Geometry check sheet. Reference: the model listing, model coordinates, mm. A direction names the side the tool comes from. Round coordinates to 2 decimals unless told otherwise and drop trailing zeros. Loops run counter-clockwise (first coordinate to the right, second up) from the corner with the lowest first, then second, coordinate; pieces in that order, holes last. Notation, with made-up numbers: (45.5, 29) - (101.5, 29) arc R21 cw to (101.5, 68) - close; hole circle Ø4 at (-11.5, 64). An arc over 180 degrees is marked (long way). Write item = value, one per line.
```python
from build123d import *

# Parameters (mm, degrees)
SKETCH1_W                = 98
SKETCH1_H                = 90
BOSS_EXTRUDE1_DEPTH      = 15
CUT_EXTRUDE1_DEPTH       = 15
CUT_EXTRUDE2_DEPTH       = 15
CUT_EXTRUDE5_DEPTH       = 100
CUT_EXTRUDE6_DEPTH       = 100
SKETCH9_R                = 9.5
CUT_EXTRUDE7_DEPTH       = 45
SKETCH10_R               = 9.5
CUT_EXTRUDE8_DEPTH       = 45
BOSS_EXTRUDE3_DEPTH      = 100
BOSS_EXTRUDE4_DEPTH      = 100
SKETCH14_W               = 54.537944566
SKETCH14_H               = 37.433727788
CUT_EXTRUDE9_DEPTH       = 100
SKETCH15_W               = 37.221464136
SKETCH15_H               = 31.979004399
CUT_EXTRUDE10_DEPTH      = 100
BOSS_EXTRUDE5_DEPTH      = 15
BOSS_EXTRUDE6_DEPTH      = 15
BOSS_EXTRUDE7_DEPTH      = 15
CUT_EXTRUDE11_DEPTH      = 100
SKETCH20_R               = 9.5
CUT_EXTRUDE12_DEPTH      = 45
SKETCH21_R               = 9.5
CUT_EXTRUDE13_DEPTH      = 100
SKETCH22_R               = 9.5
BOSS_EXTRUDE8_DEPTH      = 55
SKETCH23_R               = 9.5
CUT_EXTRUDE14_DEPTH      = 55
SKETCH24_R               = 9.5
CUT_EXTRUDE15_DEPTH      = 100
SKETCH25_R               = 9.5
BOSS_EXTRUDE10_DEPTH     = 100
SKETCH26_R               = 9.5
CUT_EXTRUDE16_DEPTH      = 100
SKETCH27_W               = 176.377882562
SKETCH27_H               = 122.842530298
SKETCH27_W_2             = 98
SKETCH27_H_2             = 90
CUT_EXTRUDE19_DEPTH      = 100
CUT_EXTRUDE19_DEPTH_BACK = 100
SKETCH28_W               = 109.510814303
SKETCH28_H               = 24.111992001
CUT_EXTRUDE20_DEPTH      = 100
SKETCH29_R               = 9.59940523
CUT_EXTRUDE21_DEPTH      = 100
SKETCH30_W               = 22
SKETCH30_H               = 32
CUT_EXTRUDE22_DEPTH      = 100
SKETCH31_W               = 16.2
SKETCH31_H               = 12
CUT_EXTRUDE23_DEPTH      = 100
CUT_EXTRUDE24_DEPTH      = 13
SKETCH33_W               = 50.373016546
SKETCH33_H               = 2
BOSS_EXTRUDE12_DEPTH     = 15
SKETCH34_W               = 20
SKETCH34_H               = 2
CUT_EXTRUDE25_DEPTH      = 5
CUT_EXTRUDE27_DEPTH      = 100
SKETCH37_W               = 14
SKETCH37_H               = 11
CUT_EXTRUDE28_DEPTH      = 13
CUT_EXTRUDE32_DEPTH      = 9.5


with BuildPart() as part:
    # Sketch1 → Boss-Extrude1 (new body)
    with BuildSketch(Plane(origin=(0, 0, 0), x_dir=(1, 0, 0), z_dir=(0, 1, 0))):
        with Locations((7.915679061, -25.165675541)):
            Rectangle(SKETCH1_W, SKETCH1_H)
    extrude(amount=BOSS_EXTRUDE1_DEPTH)

    # Sketch3 → Cut-Extrude1 (cut)
    with BuildSketch(Plane(origin=(0, 15, 0), x_dir=(1, 0, 0), z_dir=(0, 1, 0))):
        Polygon((-41.084320939, -35.165675541), (-6.084320939, -70.165675541), (-41.084320939, -70.165675541), align=None)
        Polygon((21.915679061, -70.165675541), (56.915679061, -35.165675541), (56.915679061, -70.165675541), align=None)
    extrude(amount=-CUT_EXTRUDE1_DEPTH, mode=Mode.SUBTRACT)

    # Sketch4 → Cut-Extrude2 (cut)
    with BuildSketch(Plane(origin=(0, 15, 0), x_dir=(1, 0, 0), z_dir=(0, 1, 0))):
        Polygon((-41.084320939, -35.165675541), (-32.241899351, -26.323253953), (-41.084320939, -17.480832365), align=None)
        Polygon((56.915679061, -17.480832365), (48.073257473, -26.323253953), (56.915679061, -35.165675541), align=None)
    extrude(amount=-CUT_EXTRUDE2_DEPTH, mode=Mode.SUBTRACT)

    # Sketch5 → Cut-Extrude5 (cut)
    with BuildSketch(Plane(origin=(-2.959322699, 0, -2.959322699), x_dir=(-0.707106781, 0, 0.707106781), z_dir=(-0.707106781, 0, -0.707106781))):
        Polygon((53.916889577, 0), (52.916889577, 15), (53.916889577, 15), align=None)
    extrude(amount=-CUT_EXTRUDE5_DEPTH, mode=Mode.SUBTRACT)

    # Sketch8 → Cut-Extrude6 (cut)
    with BuildSketch(Plane(origin=(10.87500176, 0, -10.87500176), x_dir=(-0.707106781, 0, -0.707106781), z_dir=(0.707106781, 0, -0.707106781))):
        Polygon((-65.11135026, 0), (-64.11135026, 15), (-65.11135026, 15), align=None)
    extrude(amount=-CUT_EXTRUDE6_DEPTH, mode=Mode.SUBTRACT)

    # Sketch9 → Cut-Extrude7 (cut)
    with BuildSketch(Plane(origin=(45.83695749, 4.321549796, 45.83695749), x_dir=(0.70866945, -0.066225327, -0.702425666), z_dir=(0.705540651, 0.066519011, 0.705540651))):
        with Locations((-0.364665022, 13.674807707)):
            Circle(SKETCH9_R)
    extrude(amount=-CUT_EXTRUDE7_DEPTH, mode=Mode.SUBTRACT)

    # Sketch10 → Cut-Extrude8 (cut)
    with BuildSketch(Plane(origin=(-37.956303558, 3.578554618, 37.956303558), x_dir=(0.70866945, 0.066225327, 0.702425666), z_dir=(-0.705540651, 0.066519011, 0.705540651))):
        with Locations((11.452044949, 13.683576238)):
            Circle(SKETCH10_R)
    extrude(amount=-CUT_EXTRUDE8_DEPTH, mode=Mode.SUBTRACT)

    # Sketch12 → Boss-Extrude3 (add)
    with BuildSketch(Plane(origin=(10.87500176, 0, -10.87500176), x_dir=(-0.707106781, 0, -0.707106781), z_dir=(0.707106781, 0, -0.707106781))):
        Polygon((-65.11135026, 0), (-64.11135026, 15), (-65.11135026, 15), align=None)
    extrude(amount=-BOSS_EXTRUDE3_DEPTH)

    # Sketch13 → Boss-Extrude4 (add)
    with BuildSketch(Plane(origin=(-2.959322699, 0, -2.959322699), x_dir=(-0.707106781, 0, 0.707106781), z_dir=(-0.707106781, 0, -0.707106781))):
        Polygon((53.916889577, 0), (52.916889577, 15), (53.916889577, 15), align=None)
    extrude(amount=-BOSS_EXTRUDE4_DEPTH)

    # Sketch14 → Cut-Extrude9 (cut)
    with BuildSketch(Plane(origin=(0, 15, 0), x_dir=(1, 0, 0), z_dir=(0, 1, 0))):
        with Locations((21.184651344, -88.882539435)):
            Rectangle(SKETCH14_W, SKETCH14_H)
    extrude(amount=-CUT_EXTRUDE9_DEPTH, mode=Mode.SUBTRACT)

    # Sketch15 → Cut-Extrude10 (cut)
    with BuildSketch(Plane(origin=(0, 15, 0), x_dir=(1, 0, 0), z_dir=(0, 1, 0))):
        with Locations((-15.067513526, -92.658393077)):
            Rectangle(SKETCH15_W, SKETCH15_H)
    extrude(amount=-CUT_EXTRUDE10_DEPTH, mode=Mode.SUBTRACT)

    # Sketch16 → Boss-Extrude5 (add)
    with BuildSketch(Plane(origin=(0, 15, 0), x_dir=(1, 0, 0), z_dir=(0, 1, 0))):
        Polygon((-6.084320939, -70.165675541), (-35.8985557, -70.165675541), (-41.084320939, -70.165675541), (-41.084320939, -35.165675541), align=None)
    extrude(amount=-BOSS_EXTRUDE5_DEPTH)

    # Sketch17 → Boss-Extrude6 (add)
    with BuildSketch(Plane(origin=(0, 15, 0), x_dir=(1, 0, 0), z_dir=(0, 1, 0))):
        Polygon((21.915679061, -70.165675541), (49.886241171, -70.165675541), (56.915679061, -70.165675541), (56.915679061, -35.165675541), align=None)
    extrude(amount=-BOSS_EXTRUDE6_DEPTH)

    # Sketch18 → Boss-Extrude7 (add)
    with BuildSketch(Plane(origin=(0, 15, 0), x_dir=(1, 0, 0), z_dir=(0, 1, 0))):
        Polygon((48.073257473, -26.323253953), (56.915679061, -17.480832365), (56.915679061, -35.165675541), align=None)
        Polygon((-41.084320939, -35.165675541), (-41.084320939, -17.480832365), (-32.241899351, -26.323253953), align=None)
    extrude(amount=-BOSS_EXTRUDE7_DEPTH)

    # Sketch19 → Cut-Extrude11 (cut)
    with BuildSketch(Plane(origin=(56.915679061, 0, 0), x_dir=(0, 0, -1), z_dir=(1, 0, 0))):
        Polygon((-70.165675541, 0), (-69.165675541, 15), (-70.165675541, 15), align=None)
    extrude(amount=-CUT_EXTRUDE11_DEPTH, mode=Mode.SUBTRACT)

    # Sketch20 → Cut-Extrude12 (cut)
    with BuildSketch(Plane(origin=(0, 4.657013863, 69.85520795), x_dir=(1, 0, 0), z_dir=(0, 0.066519011, 0.997785158))):
        with Locations((7.915679061, 13.33264869)):
            Circle(SKETCH20_R)
    extrude(amount=-CUT_EXTRUDE12_DEPTH, mode=Mode.SUBTRACT)

    # Sketch21 → Cut-Extrude13 (cut)
    with BuildSketch(Plane(origin=(14.087628182, 1.328194322, 14.087628182), x_dir=(0.70866945, -0.066225327, -0.702425666), z_dir=(0.705540651, 0.066519011, 0.705540651))):
        with Locations((2.201455665, 13.878873478)):
            Circle(SKETCH21_R)
    extrude(amount=CUT_EXTRUDE13_DEPTH, mode=Mode.SUBTRACT)

    # Sketch22 → Boss-Extrude8 (add)
    with BuildSketch(Plane(origin=(14.087628182, 1.328194322, 14.087628182), x_dir=(0.70866945, -0.066225327, -0.702425666), z_dir=(0.705540651, 0.066519011, 0.705540651))):
        with Locations((-0.364665022, 13.674807707)):
            Circle(SKETCH22_R)
    extrude(amount=BOSS_EXTRUDE8_DEPTH)

    # Sketch23 → Cut-Extrude14 (cut)
    with BuildSketch(Plane(origin=(52.892364003, 4.986739901, 52.892364003), x_dir=(0.702425666, 0.066225327, -0.70866945), z_dir=(0.705540651, 0.066519011, 0.705540651))):
        with Locations((4.020343442, 13.465005557)):
            Circle(SKETCH23_R)
    extrude(amount=-CUT_EXTRUDE14_DEPTH, mode=Mode.SUBTRACT)

    # Sketch24 → Cut-Extrude15 (cut)
    with BuildSketch(Plane(origin=(-6.20697425, 0.585199144, 6.20697425), x_dir=(0.70866945, 0.066225327, 0.702425666), z_dir=(-0.705540651, 0.066519011, 0.705540651))):
        with Locations((8.951834225, 13.883257743)):
            Circle(SKETCH24_R)
    extrude(amount=CUT_EXTRUDE15_DEPTH, mode=Mode.SUBTRACT)

    # Sketch25 → Boss-Extrude10 (add)
    with BuildSketch(Plane(origin=(-6.20697425, 0.585199144, 6.20697425), x_dir=(0.70866945, 0.066225327, 0.702425666), z_dir=(-0.705540651, 0.066519011, 0.705540651))):
        with Locations((11.452044949, 13.683576238)):
            Circle(SKETCH25_R)
    extrude(amount=BOSS_EXTRUDE10_DEPTH)

    # Sketch26 → Cut-Extrude16 (cut)
    with BuildSketch(Plane(origin=(-6.20697425, 0.585199144, 6.20697425), x_dir=(0.70866945, 0.066225327, 0.702425666), z_dir=(-0.705540651, 0.066519011, 0.705540651))):
        with Locations((8.951834225, 13.883257743)):
            Circle(SKETCH26_R)
    extrude(amount=CUT_EXTRUDE16_DEPTH, mode=Mode.SUBTRACT)

    # Sketch27 → Cut-Extrude19 (cut, two sides)
    with BuildSketch(Plane(origin=(0, 15, 0), x_dir=(1, 0, 0), z_dir=(0, 1, 0))) as cut_extrude19_sk:
        with Locations((3.867081439, -38.319377922)):
            Rectangle(SKETCH27_W, SKETCH27_H)
        with Locations((7.915679061, -25.165675541)):
            Rectangle(SKETCH27_W_2, SKETCH27_H_2, mode=Mode.SUBTRACT)
    extrude(amount=CUT_EXTRUDE19_DEPTH, mode=Mode.SUBTRACT)
    extrude(cut_extrude19_sk.sketch, amount=-CUT_EXTRUDE19_DEPTH_BACK, mode=Mode.SUBTRACT)

    # Sketch28 → Cut-Extrude20 (cut)
    with BuildSketch(Plane(origin=(0, 0, -19.834324459), x_dir=(-1, 0, 0), z_dir=(0, 0, -1))):
        with Locations((-2.16027191, 27.055996001)):
            Rectangle(SKETCH28_W, SKETCH28_H)
    extrude(amount=-CUT_EXTRUDE20_DEPTH, mode=Mode.SUBTRACT)

    # Sketch29 → Cut-Extrude21 (cut)
    with BuildSketch(Plane(origin=(0, 1.66365839, 24.954875847), x_dir=(1, 0, 0), z_dir=(0, 0.066519011, 0.997785158))):
        with Locations((7.822016096, 13.365945069)):
            Circle(SKETCH29_R)
    extrude(amount=CUT_EXTRUDE21_DEPTH, mode=Mode.SUBTRACT)

    # Sketch30 → Cut-Extrude22 (cut)
    with BuildSketch(Plane(origin=(0, 15, 0), x_dir=(1, 0, 0), z_dir=(0, 1, 0))):
        with Locations((-30.084320939, 3.834324459)):
            Rectangle(SKETCH30_W, SKETCH30_H)
        with Locations((45.915679061, 3.834324459)):
            Rectangle(SKETCH30_W, SKETCH30_H)
    extrude(amount=-CUT_EXTRUDE22_DEPTH, mode=Mode.SUBTRACT)

    # Sketch31 → Cut-Extrude23 (cut)
    with BuildSketch(Plane(origin=(34.915679061, 0, 0), x_dir=(0, 0, -1), z_dir=(1, 0, 0))):
        with Locations((3.834324459, 9)):
            Rectangle(SKETCH31_W, SKETCH31_H)
    extrude(amount=-CUT_EXTRUDE23_DEPTH, mode=Mode.SUBTRACT)

    # Sketch32 → Cut-Extrude24 (cut)
    with BuildSketch(Plane(origin=(0, 15, 0), x_dir=(1, 0, 0), z_dir=(0, 1, 0))):
        Polygon((-1.776033561, -26.490930679), (32.915679061, -26.490930679), (32.915679061, -6.265675541), (-1.776033561, -6.265675541), (-17.084320939, -6.265675541), (-17.084320939, -26.490930679), align=None)
    extrude(amount=-CUT_EXTRUDE24_DEPTH, mode=Mode.SUBTRACT)

    # Sketch33 → Boss-Extrude12 (add)
    with BuildSketch(Plane(origin=(0, 15, 0), x_dir=(1, 0, 0), z_dir=(0, 1, 0))):
        with Locations((7.729170788, -5.265675541)):
            Rectangle(SKETCH33_W, SKETCH33_H)
    extrude(amount=-BOSS_EXTRUDE12_DEPTH)

    # Sketch34 → Cut-Extrude25 (cut)
    with BuildSketch(Plane(origin=(0, 15, 0), x_dir=(1, 0, 0), z_dir=(0, 1, 0))):
        with Locations((7.915679061, -5.265675541)):
            Rectangle(SKETCH34_W, SKETCH34_H)
    extrude(amount=-CUT_EXTRUDE25_DEPTH, mode=Mode.SUBTRACT)

    # Sketch35 → Cut-Extrude27 (cut)
    with BuildSketch(Plane(origin=(56.915679061, 0, 0), x_dir=(0, 0, -1), z_dir=(1, 0, 0))):
        Polygon((-70.165675541, 0), (-62.165675541, 3), (-59.165675541, 15), (-69.165675541, 15), align=None)
    extrude(amount=-CUT_EXTRUDE27_DEPTH, mode=Mode.SUBTRACT)

    # Sketch37 → Cut-Extrude28 (cut)
    with BuildSketch(Plane(origin=(0, 15, 0), x_dir=(1, 0, 0), z_dir=(0, 1, 0))):
        with Locations((-32.084320939, -51.665675541)):
            Rectangle(SKETCH37_W, SKETCH37_H)
        with Locations((47.915679061, -51.665675541)):
            Rectangle(SKETCH37_W, SKETCH37_H)
    extrude(amount=-CUT_EXTRUDE28_DEPTH, mode=Mode.SUBTRACT)

    # Sketch38 → Cut-Extrude32 (cut)
    with BuildSketch(Plane(origin=(0, 15, 0), x_dir=(1, 0, 0), z_dir=(0, 1, 0))):
        Polygon((1.978443982, -26.490930679), (12.978443982, -26.490930679), (12.978443982, -60.585728785), (12.978443982, -67.440751443), (1.978443982, -67.440751443), (1.978443982, -60.585728785), align=None)
    extrude(amount=-CUT_EXTRUDE32_DEPTH, mode=Mode.SUBTRACT)


solid = part.part
```
(1) Section check C-C (z = -1). Enter the section's corners in (x, y), then the cut area to 3 significant figures.
Answers follow:
outline = (-19.08, 0) - (34.92, 0) - (34.92, 3) - (-19.08, 3) - close
area = 162 mm²
(2) Section check A-A (y = 4.25). Enter the section's corners in (x, z), then the cut area to 3 significant figures.
Answers follow:
outline = (-41.08, 12.17) - (-19.08, 12.17) - (-19.08, 4.27) - (34.92, 4.27) - (34.92, 12.17) - (56.92, 12.17) - (56.92, 61.85) - (-41.08, 61.85) - close; (-19.08, -19.83) - (34.92, -19.83) - (34.92, -11.93) - (-19.08, -11.93) - close; hole (-39.08, 46.17) - (-25.08, 46.17) - (-25.08, 57.17) - (-39.08, 57.17) - close; hole (-17.08, 6.27) - (32.92, 6.27) - (32.92, 26.49) - (-17.08, 26.49) - close; hole (40.92, 46.17) - (54.92, 46.17) - (54.92, 57.17) - (40.92, 57.17) - close
area = 4,400 mm²
(3) Gauge pin test, flat ends, axial feed: pin 1 (3 mm diameter, centred on x = -33, y = 5.5, fed in from +Z); pin 2 (3.5 mm diameter, centred on x = 45, z = 53.5, fed in from +Y); pin 3 (0.6 mm diameter, centred on y = 13, z = 5, fed in from -X). Record the tip position at first contact, or that the pin passes through.
Answers follow:
pin_1 = 61.92
pin_2 = 2
pin_3 = -19.08
(4) Set-up check for faces 1 (the flat face through (8, 9, 4.266)), 2 (the flat face through (-17.084, 7, 14)), 3 (the flat face through (-30, 8, 12.166)), 4 (the flat face through (12.978, 7, 48)): record each of +Z, -Z, +X, -X, +Y, -Y from which the full face is reachable in a straight line by a thin tool's end or side.
Answers follow:
face_1 = +X, -X, +Y
face_2 = +Y
face_3 = -Z, -X, +Y, -Y
face_4 = +Z, +Y
(5) Section check B-B (x = 7.5). Enter the section's corners in (y, z), then the cut area to 3 significant figures.
Answers follow:
outline = (0, -19.83) - (15, -19.83) - (15, -11.93) - (3, -11.93) - (3, 4.27) - (10, 4.27) - (10, 6.27) - (2, 6.27) - (2, 26.49) - (5.5, 26.49) - (5.5, 61.54) - (3, 62.17) - (0, 70.17) - close
area = 435 mm²
(6) Scan lines: L1, parallel to Z at x = 6, y = 7.75; L2, parallel to Z at x = 50.5, y = 5.5; L3, parallel to Z at x = 13.5, y = 6.25. Record each from-to range of solid material in increasing order. Write a range as [from, to].
Answers follow:
L1 = [-19.83, -11.93], [4.27, 6.27]
L2 = [12.17, 46.17], [57.17, 61.54]
L3 = [-19.83, -11.93], [4.27, 6.27], [26.49, 61.35]
(7) Mould release check, pull along X, two halves, no side actions. Record for faces 5 (the flat face through (-32, 2, 52)), 6 (the flat face through (8, 7, -19.834)), 7 (the flat face through (-19.084, 2.6, -3.6)): pulls with the +X half, pulls with the -X half, needs draft (parallel to the pull), parting line crosses it, or undercut.
Answers follow:
face_5 = undercut
face_6 = needs draft
face_7 = pulls with the -X half
